Build history of the part. All positions in model axes, mm. Round coordinates to 2 decimals unless told otherwise and drop trailing zeros. Write each loop counter-clockwise with the first axis right and the second up, starting at its lowest first coordinate (ties: lowest second). Pieces come first, ordered by that corner, then holes. Notation, with made-up numbers: (78, 53.5) -> (89, 53.5) arc R16 cw to (89, 82.5) -> close; hole circle Ø8 at (-23.5, 48.25). An arc over 180 degrees is marked (long way). Answer as CSV lines item,"result".
Autodesk Fusion 360 part; units mm, degrees
sketch "Sketch1" plane through (0, 0, 0) normal (0, 0, 1) x (1, 0, 0)
  line L0 (0, 0) -> (70, 0)
  line L1 (70, 0) -> (70, 150)
  line L2 (70, 150) -> (0, 150)
  line L3 (0, 150) -> (0, 0)
  circle A0 centre (22.5, 25) radius 3.3
  circle A1 centre (47.5, 25) radius 3.3
  circle A2 centre (22.5, 125) radius 3.3
  circle A3 centre (47.5, 125) radius 3.3
  line L4 (22.5, 25) -> (0, 25)
  line L5 (0, 25) -> (31, 25)
  line L6 (31, 25) -> (31, 37.5)
  line L7 (31, 37.5) -> (0, 37.5)
  line L8 (0, 37.5) -> (0, 25)
  line L9 (0, 25) -> (31, 25)
  line L10 (31, 25) -> (31, 12.5)
  line L11 (31, 12.5) -> (0, 12.5)
  line L12 (0, 12.5) -> (0, 25)
  line L13 (70, 37.5) -> (39, 37.5)
  line L14 (39, 37.5) -> (39, 12.5)
  line L15 (39, 12.5) -> (70, 12.5)
  line L16 (70, 12.5) -> (70, 37.5)
  line L17 (70, 137.5) -> (39, 137.5)
  line L18 (39, 137.5) -> (39, 112.5)
  line L19 (39, 112.5) -> (70, 112.5)
  line L20 (70, 112.5) -> (70, 137.5)
  line L21 (0, 137.5) -> (31, 137.5)
  line L22 (31, 137.5) -> (31, 112.5)
  line L23 (31, 112.5) -> (0, 112.5)
  line L24 (0, 112.5) -> (0, 137.5)
  point P0 (22.5, 25)
  point P1 (47.5, 25)
  point P2 (47.5, 125)
  point P3 (22.5, 125)
  dimension "d1" = 70
  dimension "d2" = 150
  dimension "d3" = 25
  dimension "d4" = 22.5
  dimension "d5" = 25
  dimension "d6" = 22.5
  dimension "d7" = 25
  dimension "d8" = 47.5
  dimension "d9" = 25
  dimension "d10" = 22.5
  dimension "d11" = 22.5
  dimension "d12" = 25
  dimension "d13" = 25
  dimension "d14" = 6.6
  dimension "d15" = 6.6
  dimension "d16" = 6.6
  dimension "d17" = 6.6
  dimension "d18" = 31
  dimension "d19" = 12.5
  dimension "d20" = 12.5
  dimension "d21" = 31
  dimension "d22" = 25
  dimension "d23" = 12.5
  dimension "d24" = 31
  dimension "d25" = 25
  dimension "d26" = 31
  dimension "d27" = 25
  dimension "d28" = 12.5
  dimension "d29" = 12.5
extrude "Extrude1" add sketch "Sketch1" along normal blind 25 contours L0 L1 L2 L3 L6 L7 L10 L11 L13 L14 L15 L17 L18 L19 L21 L22 L23 | L3 A0 L4 L5 L9 L10 L11 L12 | L1 L13 L14 L15 L16 | L3 A0 L4 L5 L6 L7 L8 L9 | L1 L17 L18 L19 L20 | L3 L21 L22 L23 L24
equation "d14 = 6 mm + 0.6 mm"
1. Cut at B-B, the plane y = 25. Write the cut outline in (x, z).
Results found:
outline,"(0, 0) -> (19.2, 0) -> (19.2, 25) -> (0, 25) -> close; (25.8, 0) -> (44.2, 0) -> (44.2, 25) -> (25.8, 25) -> close; (50.8, 0) -> (70, 0) -> (70, 25) -> (50.8, 25) -> close"
2. Drop a flat-ended pin along its axis: pin 1 Ø6 at (x, y) = (47.5, 25) entering from +Z. Give the stop position or say it passes through.
Results found:
pin 1,"passes through"
3. Mould opens along Y. For faces 1 (the cylindrical face through (44.881, 127.008, 12.325)), 2 (the flat face through (35, 150, 12)), 3 (the flat face through (0, 76, 12)), 4 (the cylindrical face through (25.55, 26.26, 12.32)) say: +Y half, -Y half, draft (parallel to the pull), parting line (faces both ways), or undercut.
Results found:
face 1,"undercut"
face 2,"+Y half"
face 3,"draft"
face 4,"undercut"
4. Probe line 1 along Y through (x, z) = (22.5, 9.5); line 2 along Y through (x, z) = (20, 8). List the from-to ranges inside material, lowest first.
Results found:
line 1,"y = 0 to 21.7, 28.3 to 121.7, 128.3 to 150"
line 2,"y = 0 to 22.85, 27.15 to 122.85, 127.15 to 150"
5. Cut at A-A, the plane x = 22.5. Write the cut outline in (y, z).
Results found:
outline,"(0, 0) -> (21.7, 0) -> (21.7, 25) -> (0, 25) -> close; (28.3, 0) -> (121.7, 0) -> (121.7, 25) -> (28.3, 25) -> close; (128.3, 0) -> (150, 0) -> (150, 25) -> (128.3, 25) -> close"
